Design review of the part built by this model. Coordinates are the model's own, in mm. Round coordinates to 2 decimals unless told otherwise and drop trailing zeros. Loops run counter-clockwise (first coordinate to the right, second up) from the corner with the lowest first, then second, coordinate; pieces in that order, holes last. Notation, with made-up numbers: (60.5, -8.75) - (91.5, -8.75) arc R32 cw to (91.5, 17.25) - close; hole circle Ø10 at (4.25, 78). An arc over 180 degrees is marked (long way). One line per question, with ' | ' between items. Start each with the question number.
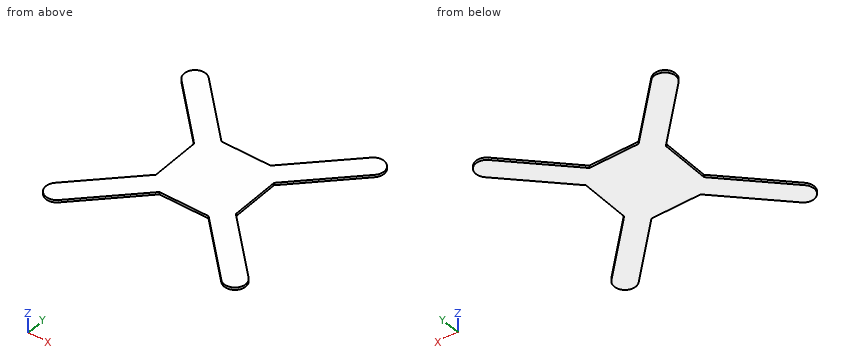
from build123d import *

# Parameters (mm, degrees)
EXTRUDE_1_DEPTH = 4


with BuildPart() as part:
    # 草图1 → 凸台-拉伸1 (new body)
    with BuildSketch(Plane.XY):
        with BuildLine():
            ThreePointArc((-132.456890143, -157.456890143), (-157.456890143, -157.456890143), (-157.456890143, -132.456890143))
            Line((-157.456890143, -132.456890143), (-65, -40))
            Line((-65, -40), (-40, -65))
            Line((-40, -65), (-132.456890143, -157.456890143))
        make_face()
        with BuildLine():
            Line((-40, 65), (-132.456890143, 157.456890143))
            ThreePointArc((-132.456890143, 157.456890143), (-157.456890143, 157.456890143), (-157.456890143, 132.456890143))
            Line((-157.456890143, 132.456890143), (-65, 40))
            Line((-65, 40), (-40, 65))
        make_face()
        Polygon((-65, 40), (-65, -40), (-40, -65), (40, -65), (65, -40), (65, 40), (40, 65), (-40, 65), align=None)
        with BuildLine():
            Line((40, -65), (132.456890143, -157.456890143))
            ThreePointArc((132.456890143, -157.456890143), (157.456890143, -157.456890143), (157.456890143, -132.456890143))
            Line((157.456890143, -132.456890143), (65, -40))
            Line((65, -40), (40, -65))
        make_face()
        with BuildLine():
            ThreePointArc((132.456890143, 157.456890143), (157.456890143, 157.456890143), (157.456890143, 132.456890143))
            Line((157.456890143, 132.456890143), (65, 40))
            Line((65, 40), (40, 65))
            Line((40, 65), (132.456890143, 157.456890143))
        make_face()
    extrude(amount=EXTRUDE_1_DEPTH)


solid = part.part
1. To check wall thickness, follow line 1 along Y through (x, z) = (36, 3.4); line 2 along Y through (x, z) = (-112, 1.6). State the ranges of each line that lie inside material, in increasing order.
2. Take a section at C-C, the plane z = 2.2. Give the boundary of the cut face in (x, y).
3. Take a section at D-D, the plane y = -51.5. Give the boundary of the cut face in (x, z).
4. Clearance check with flat-ended pins moving along their axes: P1, Ø2, axis at x = -35, z = 3, coming from the -Y side; P2, Ø2, axis at x = -90, z = 3, coming from the +Y side; P3, Ø2, axis at y = 11, z = 2.5, coming from the -X side. State where each tip first meets the part, or that it passes through.
5. Take a section at A-A, the plane y = -115.5. Give the boundary of the cut face in (x, z), then the cut area to 3 significant figures.
6. Take a section at B-B, the plane x = -96.5. Give the boundary of the cut face in (y, z).
Answer list:
1) line 1: y = -65 to 65 | line 2: y = -137 to -87, 87 to 137
2) outline: (-157.46, -132.46) arc R17.68 ccw to (-132.46, -157.46) - (-40, -65) - (40, -65) - (132.46, -157.46) arc R17.68 ccw to (157.46, -132.46) - (65, -40) - (65, 40) - (157.46, 132.46) arc R17.68 ccw to (132.46, 157.46) - (40, 65) - (-40, 65) - (-132.46, 157.46) arc R17.68 ccw to (-157.46, 132.46) - (-65, 40) - (-65, -40) - close
3) outline: (-76.5, 0) - (76.5, 0) - (76.5, 4) - (-76.5, 4) - close
4) P1: stops at y = -65 | P2: stops at y = 116 | P3: stops at x = -65
5) outline: (-140.5, 0) - (-90.5, 0) - (-90.5, 4) - (-140.5, 4) - close; (90.5, 0) - (140.5, 0) - (140.5, 4) - (90.5, 4) - close | area: 400 mm²
6) outline: (-121.5, 0) - (-71.5, 0) - (-71.5, 4) - (-121.5, 4) - close; (71.5, 0) - (121.5, 0) - (121.5, 4) - (71.5, 4) - close
